Could you check a few things on this model? Use its own coordinates, in mm. Face numbers are marked on the shaded views. A direction names the side the tool comes from. Give positions to 0.01 mm unless a question says otherwise; leave off trailing zeros. Order: outer loops, then holes, each group sorted by start corner. A loop starts at its lowest first (then second) coordinate and runs counter-clockwise, first axis right, second up. Notation, with made-up numbers: (-34, 34.25) -> (-14, 34.25) arc R14 ccw to (-14, 39.25) -> close; hole circle Ø8 at (5, -26.5). An arc over 180 degrees is marked (long way). One line per item, written item: value.
```python
from build123d import *

# Parameters (mm, degrees)
BOSS_EXTRUDE1_DEPTH = 10
SKETCH4_R           = 1.75
CUT_EXTRUDE3_DEPTH  = 10
SKETCH6_R           = 2
CUT_EXTRUDE5_DEPTH  = 2
CUT_EXTRUDE6_DEPTH  = 31.66757245
SKETCH8_W           = 5
SKETCH8_H           = 4.5
SKETCH8_W_2         = 4.5
SKETCH8_H_2         = 5
CUT_EXTRUDE7_DEPTH  = 5
FILLET1_R           = 0.5


with BuildPart() as part:
    # Sketch1 → Boss-Extrude1 (new body)
    with BuildSketch(Plane(origin=(0, 0, 0), x_dir=(1, 0, 0), z_dir=(0, 1, 0))):
        Polygon((0, 0), (20.5, 0), (20.5, -20.5), (15.5, -20.5), (15.5, -16), (4.5, -16), (4.5, -5), (0, -5), align=None)
    extrude(amount=BOSS_EXTRUDE1_DEPTH)

    # Sketch4 → Cut-Extrude3 (cut)
    with BuildSketch(Plane(origin=(0, 10, 0), x_dir=(1, 0, 0), z_dir=(0, 1, 0))):
        with Locations(Location((9.5, -11, 0), (0, 0, 270))):
            Circle(SKETCH4_R)
    extrude(amount=-CUT_EXTRUDE3_DEPTH, mode=Mode.SUBTRACT)

    # Sketch6 → Cut-Extrude5 (cut)
    with BuildSketch(Plane(origin=(0, 10, 0), x_dir=(1, 0, 0), z_dir=(0, 1, 0))):
        with Locations(Location((9.5, -11, 0), (0, 0, 270))):
            Circle(SKETCH6_R)
    extrude(amount=-CUT_EXTRUDE5_DEPTH, mode=Mode.SUBTRACT)

    # Sketch7 → Cut-Extrude6 (cut, through all)
    with BuildSketch(Plane.XZ):
        with BuildLine():
            Line((0, 8), (4.5, 8))
            ThreePointArc((4.5, 8), (6, 6.5), (4.5, 5))
            Line((4.5, 5), (0, 5))
            ThreePointArc((0, 5), (-1.5, 6.5), (0, 8))
        make_face()
        with BuildLine():
            Line((12.5, 16), (12.5, 20.5))
            ThreePointArc((12.5, 20.5), (14, 22), (15.5, 20.5))
            Line((15.5, 20.5), (15.5, 16))
            ThreePointArc((15.5, 16), (14, 14.5), (12.5, 16))
        make_face()
    extrude(amount=-CUT_EXTRUDE6_DEPTH, mode=Mode.SUBTRACT)

    # Sketch8 → Cut-Extrude7 (cut)
    with BuildSketch(Plane(origin=(0, 10, 0), x_dir=(1, 0, 0), z_dir=(0, 1, 0))):
        with Locations((18, -18.25)):
            Rectangle(SKETCH8_W, SKETCH8_H)
        with Locations((2.25, -2.5)):
            Rectangle(SKETCH8_W_2, SKETCH8_H_2)
    extrude(amount=-CUT_EXTRUDE7_DEPTH, mode=Mode.SUBTRACT)

    # Fillet1
    fillet1_edges = [part.edges().sort_by_distance(p)[0] for p in [
        (4.5, 5, 16),
        (20.5, 5, 0),
        (20.5, 2.5, 20.5),
        (15.5, 2.5, 20.5),
        (0, 2.5, 5),
        (0, 2.5, 0),
    ]]
    fillet(fillet1_edges, radius=FILLET1_R)


solid = part.part
```
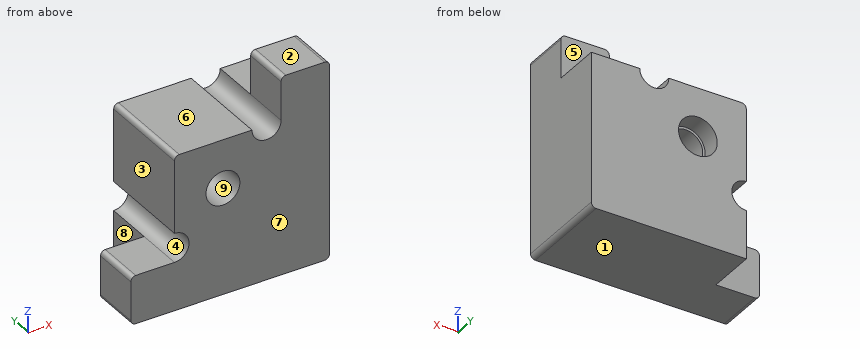
1) We'd pull the mould along Z, two halves only. Please class the marked faces 1, 2, 3 and 4: +Z half, -Z half, draft (parallel to the pull), parting line (faces both ways), or undercut.
Answer below:
face 1: -Z half
face 2: +Z half
face 3: draft
face 4: undercut
2) For P1, Ø5, axis at x = 5, y = 8, coming from the +Z side; P2, Ø3, axis at x = 1.5, y = 2.5, coming from the +Z side; P3, Ø1.5, axis at x = 5.5, z = 16.5, coming from the +Y side; P4, Ø5, axis at y = 2, z = 12.5, coming from the -X side, each with a flat end and sliding along its axis, tell me the tip position at first contact or that it passes through.
Answer below:
P1: stops at z = 16
P2: stops at z = 5
P3: stops at y = 10
P4: stops at x = 4.5
3) For the marked faces 5, 6, 7, 8 and 9, which set-ups out of +Z, -Z, +X, -X, +Y, -Y let a thin tool reach every point of the face, with its end or its side?
Answer below:
face 5: +Z, +X, -X, +Y
face 6: +Z, -X, +Y, -Y
face 7: +Z, -Z, +X, -X, -Y
face 8: +Z, -Z, -X, +Y
face 9: +Y, -Y
4) Suppose I cut it at D-D, the plane z = 2.75. Write out the boundary of the cut face in (x, y).
Answer below:
outline: (0, 0) -> (20.5, 0) -> (20.5, 10) -> (4.5, 10) -> (4.5, 5) -> (0, 5) -> close
5) Suppose I cut it at C-C, the plane x = 8.25. Write out the boundary of the cut face in (y, z), then the cut area to 3 significant figures.
Answer below:
outline: (0, 0) -> (10, 0) -> (10, 9.44) -> (8, 9.44) -> (8, 9.78) -> (0, 9.78) -> close; (0, 12.22) -> (8, 12.22) -> (8, 12.56) -> (10, 12.56) -> (10, 16) -> (0, 16) -> close
area: 134 mm2
6) If I drill on line 1 along X through (y, z) = (5, 11); line 2 along Z through (x, y) = (16.75, 9.75); line 3 along X through (y, z) = (8.55, 11), over which ranges is the centre line in solid material (lowest first)?
Answer below:
line 1: x = 4.5 to 7.75, 11.25 to 20.5
line 2: z = 0 to 16
line 3: x = 4.5 to 7.5, 11.5 to 20.5
7) Suppose I cut it at B-B, the plane y = 4.5. Write out the boundary of the cut face in (x, z).
Answer below:
outline: (0, 0.5) arc R0.5 ccw to (0.5, 0) -> (20, 0) arc R0.5 ccw to (20.5, 0.5) -> (20.5, 20) arc R0.5 ccw to (20, 20.5) -> (16, 20.5) arc R0.5 ccw to (15.5, 20) -> (15.5, 16) arc R1.5 cw to (12.5, 16) -> (5, 16) arc R0.5 ccw to (4.5, 15.5) -> (4.5, 8) arc R1.5 cw to (4.5, 5) -> (0.5, 5) arc R0.5 ccw to (0, 4.5) -> close; hole circle Ø3.5 at (9.5, 11)
8) Suppose I cut it at A-A, the plane z = 11. Write out the boundary of the cut face in (x, y).
Answer below:
outline: (4.5, 0) -> (7.75, 0) -> (7.75, 8) -> (7.5, 8) -> (7.5, 10) -> (4.5, 10) -> close; (11.25, 0) -> (20.5, 0) -> (20.5, 10) -> (11.5, 10) -> (11.5, 8) -> (11.25, 8) -> close
